Work out the finished part from the listing and answer in its coordinate system (mm). A direction names the side the tool comes from. Round coordinates to 2 decimals unless told otherwise and drop trailing zeros. Loops run counter-clockwise (first coordinate to the right, second up) from the corner with the lowest first, then second, coordinate; pieces in that order, holes last. Notation, with made-up numbers: M 47,28.5 L 72,28.5 A18 cw 72,53.5 Z; hole C 74.5,41.25 d4. An arc over 180 degrees is marked long. One line per item, written item: value.
```python
from build123d import *

# Parameters (mm, degrees)
BOSS_EXTRUDE1_DEPTH = 3.175
CUT_EXTRUDE1_DEPTH  = 72.369475764


with BuildPart() as part:
    # Sketch1 → Boss-Extrude1 (new body)
    with BuildSketch(Plane(origin=(0, 0, 0), x_dir=(1, 0, 0), z_dir=(0, 1, 0))):
        Polygon((0, 0), (13.335, 0), (13.335, -3.175), (32.385, -3.175), (32.385, 0), (45.72, 0), (45.72, 7.62), (48.895, 7.62), (48.895, 15.24), (45.72, 15.24), (45.72, 22.86), (48.895, 22.86), (48.895, 30.48), (45.72, 30.48), (45.72, 38.99662), (32.027322928, 42.858715639), (31.165424808, 39.802941329), (12.830778951, 44.974330052), (13.692677072, 48.030104361), (0, 51.8922), (0, 30.48), (-3.175, 30.48), (-3.175, 22.86), (0, 22.86), (0, 15.24), (-3.175, 15.24), (-3.175, 7.62), (0, 7.62), align=None)
    extrude(amount=BOSS_EXTRUDE1_DEPTH)

    # Sketch2 → Cut-Extrude1 (cut, through all)
    with BuildSketch(Plane(origin=(0, 3.175, 0), x_dir=(1, 0, 0), z_dir=(0, 1, 0))):
        Polygon((0, 20.4978), (3.175, 20.4978), (3.175, 21.7297), (5.461, 21.7297), (5.461, 20.4978), (10.541, 20.4978), (10.541, 17.6022), (5.461, 17.6022), (5.461, 16.3703), (3.175, 16.3703), (3.175, 17.6022), (0, 17.6022), align=None)
        Polygon((42.545, 17.6022), (45.72, 17.6022), (45.72, 20.4978), (42.545, 20.4978), (42.545, 21.7297), (40.259, 21.7297), (40.259, 20.4978), (35.179, 20.4978), (35.179, 17.6022), (40.259, 17.6022), (40.259, 16.3703), (42.545, 16.3703), align=None)
    extrude(amount=-CUT_EXTRUDE1_DEPTH, mode=Mode.SUBTRACT)


solid = part.part
```
1) Find section B-B (z = -1.5). Give the vertices of the cut face in (x, y) (3 decimals), then the cut area to 3 significant figures.
Check values:
outline: M 0,0 L 45.72,0 L 45.72,3.175 L 0,3.175 Z
area: 145 mm2
2) Find section C-C (x = 2.5). Give the vertices of the cut face in (y, z) (3 decimals).
Check values:
outline: M 0,-51.187 L 3.175,-51.187 L 3.175,-20.498 L 0,-20.498 Z; M 0,-17.602 L 3.175,-17.602 L 3.175,0 L 0,0 Z
3) The mould has two halves that part along X. Classify faces 6 (the face through (8, 2, -17.602)), 7 (the face through (4, 2, -16.37)), 8 (the face through (0, 2, -4)), 9 (the face through (35.179, 2, -19)): +X half, -X half, draft (parallel to the pull), parting line (faces both ways), or undercut.
Check values:
face 6: draft
face 7: undercut
face 8: -X half
face 9: +X half
4) Find section A-A (x = 41.5). Give the vertices of the cut face in (y, z) (3 decimals), then the cut area to 3 significant figures.
Check values:
outline: M 0,-40.187 L 3.175,-40.187 L 3.175,-21.73 L 0,-21.73 Z; M 0,-16.37 L 3.175,-16.37 L 3.175,0 L 0,0 Z
area: 111 mm2
5) Find the intervals of material crossed by probe 1 along X at (y, z) = (2.95, -2); probe 2 along X at (y, z) = (2.85, 1.5) (3 decimals); probe 3 along Z at (x, y) = (1, 1.15), in increasing order. Write a range as from..to.
Check values:
probe 1: 0..45.72
probe 2: 13.335..32.385
probe 3: -51.61..-20.5, -17.6..0
6) For faces 1 (the face through (41, 2, -16.37)), 2 (the face through (38, 2, -17.602)), 3 (the face through (45.72, 2, -35)), 4 (the face through (39, 2, 0)), 5 (the face through (31.6, 1.57, -41.35)), determine the directions among +Z, -Z, +X, -X, +Y, -Y from which every point of the face is accessible in a straight line to the end or side of a thin tool.
Check values:
face 1: +Y, -Y
face 2: +X, +Y, -Y
face 3: -Z, +X, +Y, -Y
face 4: +Z, +X, +Y, -Y
face 5: -Z, +Y, -Y
7) Each of these flat-tipped pins is pushed along its axis until it touches: pin 1 (1.6 mm diameter, centred on x = -1, y = 2, fed in from +Z); pin 2 (1 mm diameter, centred on y = 1, z = -17, fed in from +X); pin 3 (1.4 mm diameter, centred on y = 1, z = -21, fed in from -X); pin 4 (8 mm diameter, centred on x = 6.5, z = -27, fed in from -Y). Where does it stop, or does it pass through?
Check values:
pin 1: z = -7.62
pin 2: x = 45.72
pin 3: x = 0
pin 4: y = 0
8) Find section D-D (x = 16). Give the vertices of the cut face in (y, z) (3 decimals), then the cut area to 3 significant figures.
Check values:
outline: M 0,-44.08 L 3.175,-44.08 L 3.175,3.175 L 0,3.175 Z
area: 150 mm2
